Source: CAD feature listing. Evaluate the final solid. Frame: model axes, mm. Coordinates: 2 decimals unless noted, no trailing zeros. Order: outer loops, then holes, each group sorted by start corner. A loop starts at its lowest first (then second) coordinate and runs counter-clockwise, first axis right, second up.
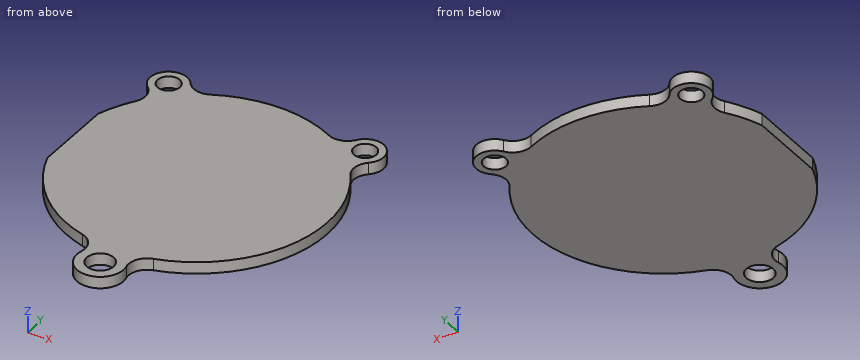
```python
from build123d import *

# Parameters (mm, degrees)
SKETCH1_R           = 1.8415
SKETCH1_R_2         = 1.524
BOSS_EXTRUDE1_DEPTH = 1.5875


with BuildPart() as part:
    # Sketch1 → Boss-Extrude1 (new body)
    with BuildSketch(Plane.XY):
        with BuildLine():
            Line((-16.984058744, -5.5245), (-16.984058744, 5.5245))
            ThreePointArc((-16.984058744, 5.5245), (-16.025769731, 7.883720963), (-14.741706386, 10.082680423))
            ThreePointArc((-14.741706386, 10.082680423), (-14.317457481, 11.828509895), (-15.154421031, 13.418289658))
            ThreePointArc((-15.154421031, 13.418289658), (-15.147832175, 17.227454165), (-11.369129629, 16.746637442))
            ThreePointArc((-11.369129629, 16.746637442), (-9.89949783, 15.713153019), (-8.113736976, 15.910550712))
            ThreePointArc((-8.113736976, 15.910550712), (0, 17.859965052), (8.113736976, 15.910550712))
            ThreePointArc((8.113736976, 15.910550712), (9.89949783, 15.713153019), (11.369129629, 16.746637442))
            ThreePointArc((11.369129629, 16.746637442), (15.147832175, 17.227454165), (15.154421031, 13.418289658))
            ThreePointArc((15.154421031, 13.418289658), (14.317457481, 11.828509895), (14.741706386, 10.082680423))
            ThreePointArc((14.741706386, 10.082680423), (16.789759308, -6.089526588), (4.850582957, -17.188664772))
            ThreePointArc((4.850582957, -17.188664772), (3.34119056, -18.362373067), (3.078011585, -20.256203417))
            ThreePointArc((3.078011585, -20.256203417), (0, -24.209965052), (-3.078011585, -20.256203417))
            ThreePointArc((-3.078011585, -20.256203417), (-3.34119056, -18.362373067), (-4.850582957, -17.188664772))
            ThreePointArc((-4.850582957, -17.188664772), (-12.377442365, -12.875452309), (-16.984058744, -5.5245))
        make_face()
        with Locations((0, -21.034965052)):
            Circle(SKETCH1_R, mode=Mode.SUBTRACT)
        with Locations((-13.470606702, 15.319965052)):
            Circle(SKETCH1_R_2, mode=Mode.SUBTRACT)
        with Locations((13.470606702, 15.319965052)):
            Circle(SKETCH1_R_2, mode=Mode.SUBTRACT)
    extrude(amount=BOSS_EXTRUDE1_DEPTH)


solid = part.part
```
1. Section query C-C on y = -13.5. Return loops of the section in (x, z).
Findings:
outline: (-11.69, 0) - (11.69, 0) - (11.69, 1.59) - (-11.69, 1.59) - close
2. Section query B-B on z = 0.9. Count the separate pieces of the cut face and the enclosed holes in it, plus the area to 3 significant figures.
Findings:
separate pieces: 1
enclosed holes: 3
area: 1,060 mm2
3. Section query A-A on x = 0. Return loops of the section in (y, z).
Findings:
outline: (-24.21, 0) - (-22.88, 0) - (-22.88, 1.59) - (-24.21, 1.59) - close; (-19.19, 0) - (17.86, 0) - (17.86, 1.59) - (-19.19, 1.59) - close
4. Section query D-D on x = -7.5. Return loops of the section in (y, z).
Findings:
outline: (-16.21, 0) - (16.21, 0) - (16.21, 1.59) - (-16.21, 1.59) - close
5. Ray query, line 1 (X direction, y = -19.5, z = 1.55); line 2 (X direction, y = 15, z = 1.35); line 3 (Y direction, x = -1.5, z = 1.2). Return the intervals inside material, ascending.
Findings:
line 1: x = -3 to -1.02, 1.02 to 3
line 2: x = -15.99 to -14.96, -11.98 to 11.98, 14.96 to 15.99
line 3: y = -23.83 to -22.1, -19.97 to 17.8
6. Pin query (flat end, axial travel): P1, Ø2.5, axis at x = 13.47, y = 15.32, coming from the +Z side. Return the tip coordinate at first contact, or that it passes through.
Findings:
P1: passes through
